Part model, mm, in its own coordinate system. Coordinates: 2 decimals unless noted, no trailing zeros. Order: outer loops, then holes, each group sorted by start corner. A loop starts at its lowest first (then second) coordinate and runs counter-clockwise, first axis right, second up. Notation, with made-up numbers: (13.5, -35.75) - (58.5, -35.75) arc R13 cw to (58.5, -14.75) - close; hole circle Ø8 at (25.25, 35). An arc over 180 degrees is marked (long way). Use a Markdown table: item, result. Add a question column.
1) Saw through at B-B on z = -197. List the corners of the cut face in (x, y) (3 decimals), then the cut area to 3 significant figures.
2) Saw through at D-D on y = -171. List the corners of the cut face in (x, z).
3) Wall check: L1, parallel to Y at x = -329, z = 102.5 (3 decimals); L2, parallel to X at y = -12.5, z = -480; L3, parallel to X at y = -115, z = -196. Give the ranges that are in metal, low to high. Write a range as [from, to].
4) Drop flat-ended pins along their axis: P1, Ø10, axis at x = -161, z = -353, coming from the +Y side; P2, Ø2.5, axis at x = -137.5, y = -2, coming from the -Z side; P3, Ø12, axis at x = -383, z = -26, coming from the -Y side (3 decimals); P4, Ø1.6, axis at y = -1, z = 133, coming from the +X side. Give the stop position or say it passes through.
5) Saw through at C-C on x = -325.5. List the corners of the cut face in (y, z) (3 decimals).
6) Saw through at A-A on x = -136. List the corners of the cut face in (y, z) (3 decimals).
```python
from build123d import *

# Parameters (mm, degrees)
F0_W     = 635
F0_H     = 762
F1_DEPTH = 3.175
F3_DEPTH = 535.94


with BuildPart() as f1:
    # F0 (on Front) → F1 (new body)
    with BuildSketch(Plane.XZ):
        with Locations((-443.691645, -2.938756)):
            Rectangle(F0_W, F0_H)
    extrude(amount=F1_DEPTH)

    # F2 (on Top) → F3 (join)
    with BuildSketch(Plane.XY):
        Polygon((0, -203.323487), (-152.235212, 0), (-152.235212, -0.024561), (-2.541544, -205.226427), align=None)
    extrude(amount=-F3_DEPTH)


solid = f1.part
```
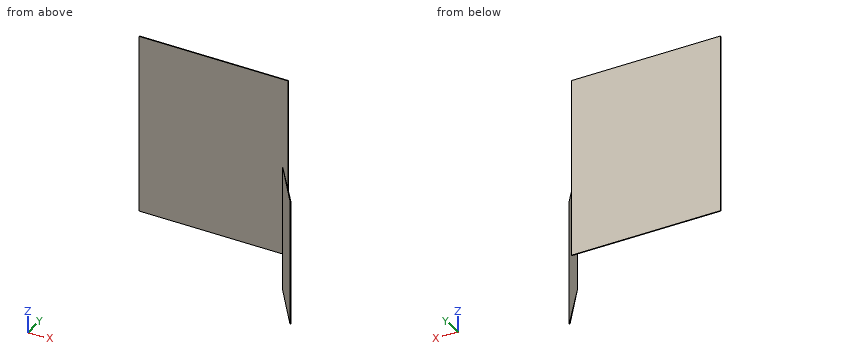
Results are:
| question | item | result |
|---|---|---|
| 1 | outline | (-761.192, -3.175) - (-149.937, -3.175) - (-2.542, -205.226) - (0, -203.323) - (-149.858, -3.175) - (-126.192, -3.175) - (-126.192, 0) - (-761.192, 0) - close |
| 1 | area | 2,420 mm2 |
| 2 | outline | (-27.51, -535.94) - (-24.2, -535.94) - (-24.2, 0) - (-27.51, 0) - close |
| 3 | L1 | [-3.175, 0] |
| 3 | L2 | [-143.13, -142.88] |
| 3 | L3 | [-68.36, -66.13] |
| 4 | P1 | y = 0 |
| 4 | P2 | z = -383.94 |
| 4 | P3 | y = -3.175 |
| 4 | P4 | x = -126.19 |
| 5 | outline | (-3.175, -383.939) - (0, -383.939) - (0, 378.061) - (-3.175, 378.061) - close |
| 6 | outline | (-22.28, -535.94) - (-21.684, -535.94) - (-21.684, 0) - (-22.28, 0) - close; (-3.175, -383.939) - (0, -383.939) - (0, 378.061) - (-3.175, 378.061) - close |
